For this review, take the finished solid that the model builds, in its own axes (mm). A direction names the side the tool comes from. Coordinates: 2 decimals unless noted, no trailing zeros. Order: outer loops, then holes, each group sorted by start corner. A loop starts at its lowest first (then second) coordinate and runs counter-clockwise, first axis right, second up. Notation, with made-up numbers: (-39, 42) -> (3, 42) arc R26 cw to (3, 67) -> close; hole circle Ø4 at (-32.75, 44.25). An arc over 180 degrees is marked (long way). Write item = value, one per line. Start each with the question number.
1) Consider section B-B on z = 5.25. Give the boundary of the cut face in (x, y), and give its area (3 significant figures).
2) Consider section D-D on y = 12. Give the boundary of the cut face in (x, z) (1 decimal).
3) Machinability: for faces 5 (the face through (3, 17, 2)), 6 (the face through (-13.203, -11.087, 2.175)), 7 (the face through (2.52, 17.19, 5.55)), which of the approach directions +Z, -Z, +X, -X, +Y, -Y give a long, thin tool a straight path to every point of the face, cutting with its end or side? Answer none if there is none.
4) Consider section A-A on y = 0. Give the boundary of the cut face in (x, z) (1 decimal).
5) Draft analysis for pull direction X (two halves, no side actions). For faces 1 (the face through (0.08, -9.07, 2.18)), 2 (the face through (-0.021, 26.175, 2.175)), 3 (the face through (-5.961, -7.196, 2.237)), 4 (the face through (16.2, -5.89, 2.18)), state which applies: +X half, -X half, draft (parallel to the pull), parting line (faces both ways), or undercut.
6) Consider section C-C on x = 0. Give the boundary of the cut face in (y, z) (1 decimal), and give its area (3 significant figures).
7) Insertion check: pin 1 Ø3 at (x, z) = (-11, 1.5) entering from -Y; pin 2 Ø3 at (x, z) = (8, 1) entering from +Y; pin 3 Ø3.5 at (y, z) = (18.5, 1.5) entering from +X; pin 4 Ø10 at (x, y) = (5.5, 16.5) entering from +Z. Each pin has a flat end and moves straight along its axis. Give the tip position at first contact, or say it passes through.
8) Wall thickness on probe 1 along Y at (x, z) = (0, 3.6); probe 2 along X at (y, z) = (0, 3.55); probe 3 along X at (y, z) = (22.5, 0.5): over which ranges is each line inside the solid? List them lowest first. Write a range as [from, to].
Autodesk Inventor part; units mm, degrees
ref_plane "YZ Plane" through (0, 0, 0) normal (1, 0, 0) x (0, 1, 0)
ref_plane "XZ Plane" through (0, 0, 0) normal (0, 1, 0) x (-1, 0, 0)
ref_plane "XY Plane" through (0, 0, 0) normal (0, 0, 1) x (1, 0, 0)
sketch "Sketch1" plane through (0, 0, 0) normal (0, 0, 1) x (1, 0, 0)
  circle A0 centre (0, 0) radius 4.0687
  arc A1 (-3, 8.5582) -> (3, 8.5582) centre (0, 0) ccw
  arc A2 (3, 26.0022) -> (-3, 26.0022) centre (0, 0) ccw
  line L0 (-3, 8.5582) -> (-3, 26.0022)
  line L1 (3, 8.5582) -> (3, 26.0022)
  dimension "d0" = 26.1747
  dimension "d2" = 6
  dimension "d3" = 5
  dimension "d4" = 8.1375
extrude "Extrusion1" add sketch "Sketch1" along normal blind 6
pattern_circular "Circular Pattern1" count 3 over 360 about axis through (0, 0, 0) along (0, 0, 1) of "Extrusion1"
fillet "Fillet1" radius 1.5875 24 edges at (-5.9116, -6.8772, 3) (5.9116, -6.8772, 3) (8.9116, -1.681, 3) (3, 8.5582, 3) (-3, 8.5582, 3) (-8.9116, -1.681, 3) (-21.0186, -15.5992, 3) (-24.0186, -10.403, 3) (-3, 26.0022, 3) (3, 26.0022, 3) (21.0186, -15.5992, 3) (24.0186, -10.403, 3) (-22.668, -13.0874, 6) (0, 26.1747, 6) (22.668, -13.0874, 6) (-13.4651, -11.2382, 6) (0, -9.0687, 6) (13.4651, -11.2382, 6) (16.4651, -6.042, 6) (7.8538, 4.5344, 6) (3, 17.2802, 6) (-3, 17.2802, 6) (-7.8538, 4.5344, 6) (-16.4651, -6.042, 6)
properties part number "ALLIGNER"
Answer sheet:
q1.outline = (-23.17, -11.66) arc R25.94 ccw to (-21.68, -14.24) arc R1.35 ccw to (-19.88, -14.66) -> (-6.95, -7.2) arc R1.83 cw to (-5, -7.28) arc R8.83 ccw to (5, -7.28) arc R1.83 cw to (6.95, -7.2) -> (19.88, -14.66) arc R1.35 ccw to (21.68, -14.24) arc R25.94 ccw to (23.17, -11.66) arc R1.35 ccw to (22.64, -9.88) -> (9.71, -2.42) arc R1.83 cw to (8.8, -0.69) arc R8.83 ccw to (3.8, 7.97) arc R1.83 cw to (2.76, 9.62) -> (2.76, 24.55) arc R1.35 ccw to (1.49, 25.89) arc R25.94 ccw to (-1.49, 25.89) arc R1.35 ccw to (-2.76, 24.55) -> (-2.76, 9.62) arc R1.83 cw to (-3.8, 7.97) arc R8.83 ccw to (-8.8, -0.69) arc R1.83 cw to (-9.71, -2.42) -> (-22.64, -9.88) arc R1.35 ccw to start; hole circle Ø8.14 at (0, 0)
q1.area = 477 mm2
q2.outline = (-3, 0) -> (3, 0) -> (3, 4.4) arc R1.6 ccw to (1.4, 6) -> (-1.4, 6) arc R1.6 ccw to (-3, 4.4) -> close
q3.face_5 = +Z, -Z, +X, +Y
q3.face_6 = +Z, -Z, -Y
q3.face_7 = +Z, +X, +Y
q4.outline = (-9.1, 0) -> (-4.1, 0) -> (-4.1, 6) -> (-7.5, 6) arc R1.6 ccw to (-9.1, 4.4) -> close; (4.1, 0) -> (9.1, 0) -> (9.1, 4.4) arc R1.6 ccw to (7.5, 6) -> (4.1, 6) -> close
q5.face_1 = undercut
q5.face_2 = parting line
q5.face_3 = undercut
q5.face_4 = +X half
q6.outline = (-9.1, 0) -> (-4.1, 0) -> (-4.1, 6) -> (-7.5, 6) arc R1.6 ccw to (-9.1, 4.4) -> close; (4.1, 0) -> (26.2, 0) -> (26.2, 4.4) arc R1.6 ccw to (24.6, 6) -> (4.1, 6) -> close
q6.area = 162 mm2
q7.pin_1 = -10.68
q7.pin_2 = 6.32
q7.pin_3 = 3
q7.pin_4 = 6
q8.probe_1 = [-9.07, -4.07], [4.07, 26.17]
q8.probe_2 = [-9.07, -4.07], [4.07, 9.07]
q8.probe_3 = [-3, 3]
